```python
from build123d import *

# Parameters (mm, degrees)
F1_DEPTH = 80
F2_R     = 2
F3_DEPTH = 25
F4_R     = 2
F5_DEPTH = 25


with BuildPart() as f1:
    # F0 (on Front) → F1 (new body)
    with BuildSketch(Plane.XZ):
        Polygon((-43.772946, 39.948631), (-46.272946, 39.948631), (-46.272946, -37.551369), (-46.272946, -40.051369), (-43.772946, -40.051369), (33.727054, -40.051369), (33.727054, -37.551369), (-43.772946, -37.551369), align=None)
    extrude(amount=F1_DEPTH)

    # F2 (on face) → F3 (cut)
    with BuildSketch(Plane(origin=(-46.272946, 0, 0), x_dir=(0, -1, 0), z_dir=(-1, 0, 0))):
        with Locations((10, 29.948631)):
            Circle(F2_R)
        with Locations((10, -10.051369)):
            Circle(F2_R)
        with Locations((30, 29.948631)):
            Circle(F2_R)
        with Locations((30, -10.051369)):
            Circle(F2_R)
        with Locations((50, 29.948631)):
            Circle(F2_R)
        with Locations((50, -10.051369)):
            Circle(F2_R)
        with Locations((70, 29.948631)):
            Circle(F2_R)
        with Locations((70, -10.051369)):
            Circle(F2_R)
        with Locations((20, 9.948631)):
            Circle(F2_R)
        with Locations((20, -30.051369)):
            Circle(F2_R)
        with Locations((40, 9.948631)):
            Circle(F2_R)
        with Locations((40, -30.051369)):
            Circle(F2_R)
        with Locations((60, 9.948631)):
            Circle(F2_R)
        with Locations((60, -30.051369)):
            Circle(F2_R)
    extrude(amount=-F3_DEPTH, mode=Mode.SUBTRACT)

    # F4 (on face) → F5 (cut)
    with BuildSketch(Plane(origin=(0, 0, -40.051369), x_dir=(1, 0, 0), z_dir=(0, 0, -1))):
        with Locations((23.727054, 70)):
            Circle(F4_R)
        with Locations((23.727054, 50)):
            Circle(F4_R)
        with Locations((23.727054, 30)):
            Circle(F4_R)
        with Locations((23.727054, 10)):
            Circle(F4_R)
        with Locations((-16.272946, 70)):
            Circle(F4_R)
        with Locations((-16.272946, 50)):
            Circle(F4_R)
        with Locations((-16.272946, 30)):
            Circle(F4_R)
        with Locations((-16.272946, 10)):
            Circle(F4_R)
        with Locations((3.727054, 60)):
            Circle(F4_R)
        with Locations((3.727054, 40)):
            Circle(F4_R)
        with Locations((3.727054, 20)):
            Circle(F4_R)
        with Locations((-36.272946, 60)):
            Circle(F4_R)
        with Locations((-36.272946, 40)):
            Circle(F4_R)
        with Locations((-36.272946, 20)):
            Circle(F4_R)
    extrude(amount=-F5_DEPTH, mode=Mode.SUBTRACT)


solid = f1.part
```
Geometry: final body of the model. Coordinates: model frame, mm. A direction names the side the tool comes from. Coordinates: 2 decimals unless noted, no trailing zeros. Order: outer loops, then holes, each group sorted by start corner. A loop starts at its lowest first (then second) coordinate and runs counter-clockwise, first axis right, second up. Notation, with made-up numbers: (-8.5, 37) -> (46.5, 37) arc R22 ccw to (46.5, 43) -> close; hole circle Ø7 at (-8, 80.5). An arc over 180 degrees is marked (long way). Write each question's results on one line, items separated by ' | '. Start each with the question number.
1) First-contact query: pin 1 (1 mm diameter, centred on x = -10.5, y = -62.5, fed in from +Z); pin 2 (6.5 mm diameter, centred on y = -70, z = -10.05, fed in from +X); pin 3 (5 mm diameter, centred on x = 23.73, y = -70, fed in from -Z). Flat tips, straight axial feed; report the tip coordinate or a pass-through.
2) Material intervals for line 1 along Z through (x, y) = (-45.3, -40); line 2 along Z through (x, y) = (-44.5, -10); line 3 along X through (y, z) = (-60, -39.3), sorted ascending.
3) Set-up query: faces 1 (the flat face through (-43.773, -39, 1)), 2 (the flat face through (-24, -80, -38)). Return all of +Z, -Z, +X, -X, +Y, -Y with unobstructed straight access to the full face (end or side cutting, diameter ignored); none if empty.
4) Mould query, pull axis Z, two halves, no side actions, for faces 3 (the cylindrical face through (-37.7, -61.4, -38.8)), 4 (the flat face through (-4, -39, -37.551)), 5 (the cylindrical face through (-45.04, -31.847, -10.817)). Classes: released by +Z, released by -Z, zero draft, split by the parting line, or undercut.
5) Cut plane A-A, the plane y = -40. Output: boundary loops of the cut face in (x, z), and give its area (3 significant figures).
6) Cut plane B-B, the plane x = -37. Output: boundary loops of the cut face in (y, z), and give its area (3 significant figures).
7) Cut plane D-D, the plane x = -12.5. Output: boundary loops of the cut face in (y, z).
8) Cut plane C-C, the plane z = -14. Output: boundary loops of the cut face in (x, y).
Checks:
1) pin 1: z = -37.55 | pin 2: x = -43.77 | pin 3: z = -40.05
2) line 1: -40.05 to -32.05, -28.05 to 7.95, 11.95 to 39.95 | line 2: -40.05 to -12.05, -8.05 to 27.95, 31.95 to 39.95 | line 3: -46.27 to -38.27, -34.27 to 1.73, 5.73 to 33.73
3) face 1: +Z, +X, +Y, -Y | face 2: +Z, -Z, +X, -X, -Y
4) face 3: zero draft | face 4: released by +Z | face 5: undercut
5) outline: (-46.27, -40.05) -> (-38.27, -40.05) -> (-38.27, -37.55) -> (-43.77, -37.55) -> (-43.77, -32.05) -> (-46.27, -32.05) -> close; (-46.27, -28.05) -> (-43.77, -28.05) -> (-43.77, 7.95) -> (-46.27, 7.95) -> close; (-46.27, 11.95) -> (-43.77, 11.95) -> (-43.77, 39.95) -> (-46.27, 39.95) -> close; (-34.27, -40.05) -> (1.73, -40.05) -> (1.73, -37.55) -> (-34.27, -37.55) -> close; (5.73, -40.05) -> (33.73, -40.05) -> (33.73, -37.55) -> (5.73, -37.55) -> close | area: 354 mm^2
6) outline: (-80, -40.05) -> (-61.86, -40.05) -> (-61.86, -37.55) -> (-80, -37.55) -> close; (-58.14, -40.05) -> (-41.86, -40.05) -> (-41.86, -37.55) -> (-58.14, -37.55) -> close; (-38.14, -40.05) -> (-21.86, -40.05) -> (-21.86, -37.55) -> (-38.14, -37.55) -> close; (-18.14, -40.05) -> (0, -40.05) -> (0, -37.55) -> (-18.14, -37.55) -> close | area: 172 mm^2
7) outline: (-80, -40.05) -> (0, -40.05) -> (0, -37.55) -> (-80, -37.55) -> close
8) outline: (-46.27, -80) -> (-43.77, -80) -> (-43.77, 0) -> (-46.27, 0) -> close
